from build123d import *

# Parameters (mm, degrees)
SKETCH1_W           = 31.75
SKETCH1_H           = 28.575
BOSS_EXTRUDE1_DEPTH = 9.525
SKETCH2_R           = 6.35
CUT_EXTRUDE1_DEPTH  = 35.048081811
SKETCH3_R           = 4.7625
CUT_EXTRUDE2_DEPTH  = 37.095993978
BOSS_EXTRUDE2_START = 1.5875
SKETCH4_R           = 6.35
SKETCH4_R_2         = 4.7625
BOSS_EXTRUDE2_DEPTH = 1.5875


with BuildPart() as part:
    # Sketch1 → Boss-Extrude1 (new, symmetric)
    with BuildSketch(Plane.XY):
        Rectangle(SKETCH1_W, SKETCH1_H)
    extrude(amount=BOSS_EXTRUDE1_DEPTH, both=True)

    # Sketch2 → Cut-Extrude1 (cut, through all)
    with BuildSketch(Plane.XZ.offset(14.2875)):
        with Locations(Location((0, 0, 0), (0, 0, 270))):
            Circle(SKETCH2_R)
    extrude(amount=-CUT_EXTRUDE1_DEPTH, mode=Mode.SUBTRACT)

    # Sketch3 → Cut-Extrude2 (cut, through all)
    with BuildSketch(Plane.ZY.offset(15.875)):
        Circle(SKETCH3_R)
    extrude(amount=-CUT_EXTRUDE2_DEPTH, mode=Mode.SUBTRACT)

    # Sketch4 → Boss-Extrude2 (add)
    with BuildSketch(Plane.ZY.offset(15.875).offset(BOSS_EXTRUDE2_START)):
        with Locations(Location((0, 0, 0), (0, 0, 180))):
            Circle(SKETCH4_R)
        Circle(SKETCH4_R_2, mode=Mode.SUBTRACT)
    boss_extrude2 = extrude(amount=-BOSS_EXTRUDE2_DEPTH)

    # Mirror1: Boss-Extrude2 across plane
    add(boss_extrude2.mirror(Plane(origin=(0, 0, 0), x_dir=(0, 0, 1), z_dir=(1, 0, 0))))


solid = part.part
Verification items for the finished model (mm, model axes). A direction names the side the tool comes from. Coordinates: 2 decimals unless noted, no trailing zeros. Order: outer loops, then holes, each group sorted by start corner. A loop starts at its lowest first (then second) coordinate and runs counter-clockwise, first axis right, second up. Notation, with made-up numbers: M -37,-15 L 19,-15 A28 ccw 19,23 Z; hole C 32,45.25 d10. An arc over 180 degrees is marked long. One line per item, written item: value. Start each with the question number.
Item 1: Sectioned sample at A-A (z = 0). Count the separate pieces of the cut face and the enclosed holes in it, then the cut area to 3 significant figures.
Item 2: Mould release check, pull along Y, two halves, no side actions. Record for faces 1 (the cylindrical face through (-16.68, 5.634, -2.93)), 2 (the cylindrical face through (10.924, 1.431, 4.543)), 3 (the cylindrical face through (-10.924, 1.431, 4.543)), 4 (the flat face through (-0.2, -14.288, 6.5)): released by +Y, released by -Y, zero draft, split by the parting line, or undercut.
Item 3: Sectioned sample at C-C (y = 10.75). Enter the section's corners in (x, z) (3 decimals), then the cut area to 3 significant figures.
Item 4: Scan lines: probe 1 along Y at (x, z) = (-12.5, 0); probe 2 along X at (y, z) = (6.25, 0); probe 3 along Z at (x, y) = (9.5, 0) (1 decimal). Record each from-to range of solid material in increasing order.
Item 5: Access from +Z, -Z, +X, -X, +Y, -Y to the whole of each face (thin tool, end or side, straight path). Record for faces 5 (the flat face through (17.462, -5, -1)), 6 (the flat face through (15.875, -0.2, 6.5)), 7 (the flat face through (-15.875, -0.2, 6.5)).
Item 6: Sectioned sample at D-D (x = 7.5). Enter the section's corners in (y, z) (1 decimal).
Conclusion:
1. separate pieces: 4
1. enclosed holes: 0
1. area: 373 mm^2
2. face 1: split by the parting line
2. face 2: undercut
2. face 3: undercut
2. face 4: released by -Y
3. outline: M -15.875,-9.525 L 15.875,-9.525 L 15.875,9.525 L -15.875,9.525 Z; hole C 0,0 d12.7
3. area: 478 mm^2
4. probe 1: y = -14.29 to -4.76, 4.76 to 14.29
4. probe 2: x = -17.46 to -6.35, 6.35 to 17.46
4. probe 3: z = -9.5 to -4.8, 4.8 to 9.5
5. face 5: +Z, -Z, +X, +Y, -Y
5. face 6: +X
5. face 7: -X
6. outline: M -14.3,-9.5 L 14.3,-9.5 L 14.3,9.5 L -14.3,9.5 Z; hole C 0,0 d9.5
